```python
from build123d import *

# Parameters (mm, degrees)
SKETCH1_W                                        = 15
SKETCH1_H                                        = 130
SKETCH1_H_2                                      = 10
BOSS_EXTRUDE1_DEPTH                              = 50.8
CBORE_FOR_1_4_SOCKET_HEAD_CAP_SCREW1_D           = 6.7564
CBORE_FOR_1_4_SOCKET_HEAD_CAP_SCREW1_CBORE_D     = 11.1125
CBORE_FOR_1_4_SOCKET_HEAD_CAP_SCREW1_CBORE_DEPTH = 6.35
F_8_CLEARANCE_HOLE2_D                            = 4.9149
LPATTERN1_COUNT                                  = 3
LPATTERN1_PITCH                                  = 20
SKETCH10_W                                       = 72.8
SKETCH10_H                                       = 25.2
CUT_EXTRUDE1_DEPTH                               = 2
SKETCH13_W                                       = 15
SKETCH13_H                                       = 5.4
BOSS_EXTRUDE2_DEPTH                              = 10
DRAFT1_ANGLE                                     = 60


with BuildPart() as part:
    # Sketch1 → Boss-Extrude1 (new body)
    with BuildSketch(Plane(origin=(0, 0, 0), x_dir=(1, 0, 0), z_dir=(0, 1, 0))):
        with Locations((-75.402654867, 8.513274336)):
            Rectangle(SKETCH1_W, SKETCH1_H)
        with Locations((-90.402654867, -51.486725664)):
            Rectangle(SKETCH1_W, SKETCH1_H_2)
    extrude(amount=BOSS_EXTRUDE1_DEPTH)

    # CBORE for 1/4 Socket Head Cap Screw1 (through all)
    with Locations(Plane(origin=(0, 0, 46.486725664), x_dir=(-1, 0, 0), z_dir=(0, 0, -1))):
        with Locations((90.402654867, 12.7), (90.402654867, 38.1)):
            CounterBoreHole(CBORE_FOR_1_4_SOCKET_HEAD_CAP_SCREW1_D / 2, CBORE_FOR_1_4_SOCKET_HEAD_CAP_SCREW1_CBORE_D / 2, CBORE_FOR_1_4_SOCKET_HEAD_CAP_SCREW1_CBORE_DEPTH)

    # #8 Clearance Hole2 (through all)
    with Locations(Plane(origin=(-67.902654867, 0, 0), x_dir=(0, 0, -1), z_dir=(1, 0, 0))):
        with Locations((63.513274336, 25.4), (53.513274336, 25.4)):
            f_8_clearance_hole2 = Hole(F_8_CLEARANCE_HOLE2_D / 2)

    # LPattern1: #8 Clearance Hole2 ×3
    with Locations(*[(0, 0, i * LPATTERN1_PITCH) for i in range(1, LPATTERN1_COUNT)]):
        add(f_8_clearance_hole2, mode=Mode.SUBTRACT)

    # Sketch10 → Cut-Extrude1 (cut)
    with BuildSketch(Plane(origin=(-67.902654867, 0, 0), x_dir=(0, 0, -1), z_dir=(1, 0, 0))):
        with Locations((37.113274336, 25.4)):
            Rectangle(SKETCH10_W, SKETCH10_H)
    extrude(amount=-CUT_EXTRUDE1_DEPTH, mode=Mode.SUBTRACT)

    # Sketch13 → Boss-Extrude2 (add)
    with BuildSketch(Plane(origin=(0, 0, 46.486725664), x_dir=(-1, 0, 0), z_dir=(0, 0, -1))):
        with Locations((90.402654867, 25.4)):
            Rectangle(SKETCH13_W, SKETCH13_H)
    extrude(amount=BOSS_EXTRUDE2_DEPTH)

    # Draft1
    draft1_faces = [part.faces().sort_by_distance(p)[0] for p in [
        (-90.402654867, 25.4, 36.486725664),
    ]]
    draft(draft1_faces, Plane(origin=(-97.902654867, 50.8, 0), x_dir=(0, 0, -1), z_dir=(-1, 0, 0)), DRAFT1_ANGLE)


solid = part.part
```
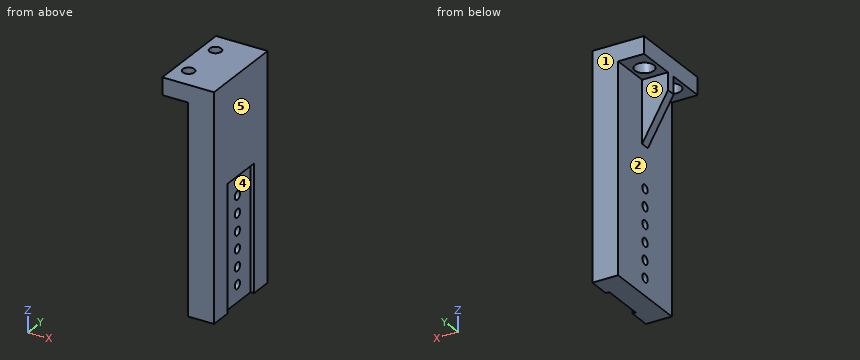
Input: part model. Units: mm. Frame: model coordinates. Face numbers are marked on the shaded views. A direction names the side the tool comes from. Give positions to 0.01 mm unless a question says otherwise; leave off trailing zeros. Order: outer loops, then holes, each group sorted by start corner. A loop starts at its lowest first (then second) coordinate and runs counter-clockwise, first axis right, second up. Notation, with made-up numbers: M 77,-27.5 L 107,-27.5 A15 cw 107,-12.5 Z; hole C 89.5,84 d2. An arc over 180 degrees is marked long. One line per question, with ' | ' between items. Start each with the question number.
1. Section query D-D (z = 25). Return the cut outline in (x, y), and give its area (3 significant figures).
2. Section query A-A (y = 25.4). Count the separate pieces of the cut face and the enclosed holes in it, and give its area (3 significant figures).
3. Section query C-C (y = 36.5). Return the cut outline in (x, z), and give its area (3 significant figures).
4. Pull-direction query (Y, two-part tool) for the marked faces 3, 4 and 5; classes: released by +Y, released by -Y, zero draft, split by the parting line, or undercut.
5. Section query B-B (x = -72). Return the cut outline in (y, z).
6. First-contact query: pin 1 Ø5.5 at (x, y) = (-92.5, 37) entering from -Z; pin 2 Ø4.5 at (y, z) = (25.4, -63.51) entering from -X; pin 3 Ø5.5 at (y, z) = (25.4, -23.51) entering from -X; pin 4 Ø4 at (x, z) = (-72, 34) entering from -Y. Flat tips, straight axial feed; report the tip coordinate or a pass-through.
7. Access query for the marked faces 1 and 2. Directions: +Z, -Z, +X, -X, +Y, -Y. A direction counts if a zero-diameter tool reaches every point of the face in a straight line with its end or side. Return the directions, or none.
8. Material intervals for probe 1 along X at (y, z) = (38, 55); probe 2 along Z at (x, y) = (-86.5, 14); probe 3 along Z at (x, y) = (-83.5, 15.5), sorted ascending. Write a range as [from, to].
Here are the results:
1) outline: M -91.27,22.7 L -82.9,22.7 L -82.9,0 L -67.9,0 L -67.9,50.8 L -82.9,50.8 L -82.9,28.1 L -91.27,28.1 Z | area: 807 mm²
2) separate pieces: 7 | enclosed holes: 0 | area: 1,920 mm²
3) outline: M -97.9,46.49 L -95.72,46.49 L -95.72,52.84 L -93.38,52.84 L -93.38,56.49 L -97.9,56.49 Z; M -87.43,52.84 L -85.08,52.84 L -85.08,46.49 L -82.9,46.49 L -82.9,-73.51 L -69.9,-73.51 L -69.9,-0.71 L -67.9,-0.71 L -67.9,56.49 L -87.43,56.49 Z | area: 1,870 mm²
4) face 3: released by +Y | face 4: undercut | face 5: zero draft
5) outline: M 0,-73.51 L 50.8,-73.51 L 50.8,56.49 L 0,56.49 Z; hole C 25.4,-63.51 d4.91; hole C 25.4,-53.51 d4.91; hole C 25.4,-43.51 d4.91; hole C 25.4,-33.51 d4.91; hole C 25.4,-23.51 d4.91; hole C 25.4,-13.51 d4.91
6) pin 1: z = 52.84 | pin 2: through | pin 3: x = -82.9 | pin 4: y = 0
7) face 1: +Z, -Z, +X, -X, +Y | face 2: -Z, -X
8) probe 1: [-97.9, -93.78], [-87.03, -67.9] | probe 2: [52.84, 56.49] | probe 3: [46.49, 56.49]
